Build history of the part. All positions in model axes, mm. A direction names the side the tool comes from. Give positions to 0.01 mm unless a question says otherwise; leave off trailing zeros. Order: outer loops, then holes, each group sorted by start corner. A loop starts at its lowest first (then second) coordinate and runs counter-clockwise, first axis right, second up. Notation, with made-up numbers: M 34,12 L 55,12 A16 ccw 55,21 Z; hole C 23,62 d9. An arc over 180 degrees is marked long. Answer as CSV lines item,"result".
from build123d import *

# Parameters (mm, degrees)
SKETCH2_W           = 203.2
SKETCH2_H           = 101.6
BOSS_EXTRUDE1_DEPTH = 31.75
SKETCH3_W           = 92.020686849
SKETCH3_H           = 101.6
CUT_EXTRUDE1_DEPTH  = 12.7
SKETCH4_R           = 12.7
SKETCH4_W           = 60.96
SKETCH4_H           = 38.1
BOSS_EXTRUDE2_DEPTH = 12.7
SKETCH6_R           = 15.875
SKETCH6_W           = 44.45
SKETCH6_H           = 50.8
CUT_EXTRUDE2_DEPTH  = 12.7
BOSS_EXTRUDE3_DEPTH = 12.7


with BuildPart() as part:
    # Sketch2 → Boss-Extrude1 (new body)
    with BuildSketch(Plane.XY):
        Rectangle(SKETCH2_W, SKETCH2_H)
    extrude(amount=BOSS_EXTRUDE1_DEPTH)

    # Sketch3 → Cut-Extrude1 (cut)
    with BuildSketch(Plane.XY.offset(31.75)):
        with Locations((55.589656576, 0)):
            Rectangle(SKETCH3_W, SKETCH3_H)
    extrude(amount=-CUT_EXTRUDE1_DEPTH, mode=Mode.SUBTRACT)

    # Sketch4 → Boss-Extrude2 (add)
    with BuildSketch(Plane.XY.offset(19.05)):
        with Locations(Location((83.82, 30.48, 0), (0, 0, 180))):  # turned: the seam where the file's is
            Circle(SKETCH4_R)
        with Locations((60.96, -26.67)):
            Rectangle(SKETCH4_W, SKETCH4_H)
    extrude(amount=BOSS_EXTRUDE2_DEPTH)

    # Sketch6 → Cut-Extrude2 (cut)
    with BuildSketch(Plane.XY.offset(31.75)):
        with Locations((-75.387587267, -5.436604851)):
            Circle(SKETCH6_R)
        with BuildLine():
            Line((-87.710558262, -30.1625), (-3.261962911, -30.1625))
            ThreePointArc((-3.261962911, -30.1625), (4.675537089, -38.1), (-3.261962911, -46.0375))
            Line((-3.261962911, -46.0375), (-87.710558262, -46.0375))
            ThreePointArc((-87.710558262, -46.0375), (-95.648058262, -38.1), (-87.710558262, -30.1625))
        make_face()
        with Locations((-22.225, 17.78)):
            Rectangle(SKETCH6_W, SKETCH6_H)
    extrude(amount=-CUT_EXTRUDE2_DEPTH, mode=Mode.SUBTRACT)

    # Sketch7 → Boss-Extrude3 (add)
    with BuildSketch(Plane.XY.offset(19.05)):
        Polygon((39.106813151, 46.977783942), (24.819313151, 38.728891971), (24.819313151, 22.231108029), (39.106813151, 13.982216058), (53.394313151, 22.231108029), (53.394313151, 38.728891971), align=None)
    extrude(amount=BOSS_EXTRUDE3_DEPTH)


solid = part.part
Item 1: Band-saw the part on C-C (y = 30.48). Give the cut face in (x, z).
Geometry says:
outline,"M -101.6,0 L 101.6,0 L 101.6,19.05 L 96.52,19.05 L 96.52,31.75 L 71.12,31.75 L 71.12,19.05 L 53.39,19.05 L 53.39,31.75 L 24.82,31.75 L 24.82,19.05 L 9.58,19.05 L 9.58,31.75 L 0,31.75 L 0,19.05 L -44.45,19.05 L -44.45,31.75 L -101.6,31.75 Z"
Item 2: 3-axis set-ups, long thin cutter, end or side, ignore diameter. For faces 1 (the flat face through (46.15, 18.05, 25.31)), 2 (the flat face through (61, -45.72, 25)), 3 (the flat face through (30.48, -27, 25)), 4 (the flat face through (46, 43, 25)): which of +Z, -Z, +X, -X, +Y, -Y reach the whole face in a straight line?
Geometry says:
face 1,"+Z"
face 2,"+Z, +X, -Y"
face 3,"+Z, -Y"
face 4,"+Z, +Y"
Item 3: Band-saw the part on D-D (x = -67). Give the cut face in (y, z), and give its area (3 significant figures).
Geometry says:
outline,"M -50.8,0 L 50.8,0 L 50.8,31.75 L 8.04,31.75 L 8.04,19.05 L -18.91,19.05 L -18.91,31.75 L -30.16,31.75 L -30.16,19.05 L -46.04,19.05 L -46.04,31.75 L -50.8,31.75 Z"
area,"2,680 mm2"
Item 4: Drop flat-ended pins along their axis: pin 1 (4 mm diameter, centred on y = 9, z = 25.5, fed in from +X); pin 2 (6.5 mm diameter, centred on x = 75, z = 23.5, fed in from +Y); pin 3 (12 mm diameter, centred on x = -44, y = -37, fed in from +Z). Give the stop position or say it passes through.
Geometry says:
pin 1,"stops at x = 9.58"
pin 2,"stops at y = 41.89"
pin 3,"stops at z = 19.05"
Item 5: Probe line 1 along Y through (x, z) = (-15.5, 22); line 2 along X through (y, z) = (-22.5, 22); line 3 along X through (y, z) = (-18.5, 29). List the from-to ranges inside material, lowest first. Write a range as from..to.
Geometry says:
line 1,"y = -50.8..-46.04, -30.16..-7.62, 43.18..50.8"
line 2,"x = -101.6..9.58, 30.48..91.44"
line 3,"x = -101.6..-84.41, -66.37..9.58, 30.48..91.44"
Item 6: Pull direction X, two halves, no side cores. Call faces 5 (the flat face through (-47, 12, 31.75)), 6 (the flat face through (-45, -38, 19.05)), 7 (the flat face through (91.44, -27, 25)): released by +X, released by -X, zero draft, split by the parting line, or undercut.
Geometry says:
face 5,"zero draft"
face 6,"undercut"
face 7,"released by +X"
Item 7: Band-saw the part on A-A (y = -38.1). Give the cut face in (x, z), and give its area (3 significant figures).
Geometry says:
outline,"M -101.6,0 L 101.6,0 L 101.6,19.05 L 91.44,19.05 L 91.44,31.75 L 30.48,31.75 L 30.48,19.05 L 9.58,19.05 L 9.58,31.75 L 4.68,31.75 L 4.68,19.05 L -95.65,19.05 L -95.65,31.75 L -101.6,31.75 Z"
area,"4,780 mm2"
Item 8: Band-saw the part on B-B (x = 83.82). Give the cut face in (y, z), and give its area (3 significant figures).
Geometry says:
outline,"M -50.8,0 L 50.8,0 L 50.8,19.05 L 43.18,19.05 L 43.18,31.75 L 17.78,31.75 L 17.78,19.05 L -7.62,19.05 L -7.62,31.75 L -45.72,31.75 L -45.72,19.05 L -50.8,19.05 Z"
area,"2,740 mm2"
